Input: part model. Units: mm. Frame: model coordinates. A direction names the side the tool comes from. Round coordinates to 2 decimals unless told otherwise and drop trailing zeros. Loops run counter-clockwise (first coordinate to the right, second up) from the corner with the lowest first, then second, coordinate; pieces in that order, holes last. Notation, with made-up numbers: (29.25, -13) -> (84.25, -13) arc R24 ccw to (84.25, 16) -> close; hole circle Ø8 at (67.5, 67). An arc over 180 degrees is marked (long way). One line per question, with ' | ' between items. Start each with the question number.
Q1. Cut plane B-B on x = 0. Return loops of the section in (y, z), and give its area (3 significant figures).
Q2. Material intervals for L1, parallel to Z at x = 0, y = -16; L2, parallel to Y at x = 1.5, z = 4.5; L3, parallel to Z at x = 0, y = -3.55, sorted ascending.
Q3. Cut plane A-A on z = 0. Return loops of the section in (x, y).
Q4. Cut plane C-C on y = -10.5. Return loops of the section in (x, z), and give its area (3 significant figures).
Q5. Access query for faces 5 (the face through (1, -60, -6)), 6 (the face through (-2, -5, -4)). Directions: +Z, -Z, +X, -X, +Y, -Y. A direction counts if a zero-diameter tool reaches every point of the face in a straight line with its end or side. Return the directions, or none.
Q6. Contact query for flat-ended pins moving along their axis: P1, Ø7.5, axis at x = 0, z = 0, coming from the -Y side; P2, Ø3, axis at y = -36, z = 2, coming from the -X side; P3, Ø2, axis at x = 6, y = -27, coming from the -Z side. Output: stop coordinate, or through.
Q7. Mould query, pull axis Z, two halves, no side actions, for faces 1 (the face through (-7.493, -29.583, 0.33)), 2 (the face through (0, 0, -5)), 3 (the face through (-1.19, -32.02, -5.37)), 4 (the face through (-0.534, -2.566, 4.065)). Classes: pulls with the +Z half, pulls with the -Z half, needs draft (parallel to the pull), parting line crosses it, or undercut.
from build123d import *

# Parameters (mm, degrees)
F0_R     = 7.5
F0_R_2   = 5.5
F1_DEPTH = 60
F0_R_3   = 4.1
F2_DEPTH = 5
F3_SIZE  = 0.2


with BuildPart() as f1:
    # F0 (on Front) → F1 (new body)
    with BuildSketch(Plane.XZ):
        Circle(F0_R)
        Circle(F0_R_2, mode=Mode.SUBTRACT)
    extrude(amount=F1_DEPTH)

    # F0 (on Front) → F2 (join)
    with BuildSketch(Plane.XZ):
        Circle(F0_R_2)
        Circle(F0_R_3, mode=Mode.SUBTRACT)
    extrude(amount=F2_DEPTH)

    # F3
    f3_edges = [f1.edges().sort_by_distance(p)[0] for p in [
        (-7.5, 0, 0),
        (-4.1, 0, 0),
        (-7.5, -60, 0),
        (-5.5, -60, 0),
    ]]
    chamfer(f3_edges, length=F3_SIZE)


solid = f1.part
Results:
1) outline: (-60, -7.3) -> (-59.8, -7.5) -> (-0.2, -7.5) -> (0, -7.3) -> (0, -4.3) -> (-0.2, -4.1) -> (-5, -4.1) -> (-5, -5.5) -> (-59.8, -5.5) -> (-60, -5.7) -> close; (-60, 5.7) -> (-59.8, 5.5) -> (-5, 5.5) -> (-5, 4.1) -> (-0.2, 4.1) -> (0, 4.3) -> (0, 7.3) -> (-0.2, 7.5) -> (-59.8, 7.5) -> (-60, 7.3) -> close | area: 254 mm^2
2) L1: -7.5 to -5.5, 5.5 to 7.5 | L2: -5 to 0 | L3: -7.5 to -4.1, 4.1 to 7.5
3) outline: (-7.5, -59.8) -> (-7.3, -60) -> (-5.7, -60) -> (-5.5, -59.8) -> (-5.5, -5) -> (-4.1, -5) -> (-4.1, -0.2) -> (-4.3, 0) -> (-7.3, 0) -> (-7.5, -0.2) -> close; (4.1, -5) -> (5.5, -5) -> (5.5, -59.8) -> (5.7, -60) -> (7.3, -60) -> (7.5, -59.8) -> (7.5, -0.2) -> (7.3, 0) -> (4.3, 0) -> (4.1, -0.2) -> close
4) outline: circle Ø15 at (0, 0); hole circle Ø11 at (0, 0) | area: 81.7 mm^2
5) face 5: +Z, -Z, +X, -X, -Y | face 6: -Y
6) P1: through | P2: x = -7.48 | P3: z = -5.59
7) face 1: parting line crosses it | face 2: needs draft | face 3: undercut | face 4: undercut
